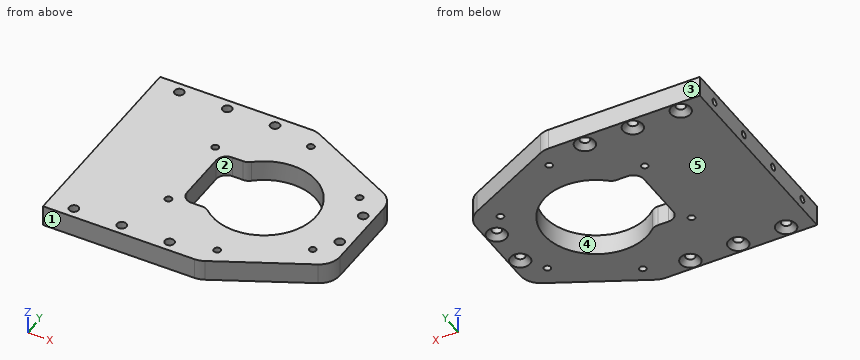
```python
from build123d import *

# Parameters (mm, degrees)
EXTRUDE1_DEPTH                                  = 10
CUT_EXTRUDE1_DEPTH                              = 20
SKETCH3_R                                       = 1.65
CUT_EXTRUDE2_DEPTH                              = 10
SKETCH4_R                                       = 1.65
CUT_EXTRUDE3_DEPTH                              = 15
FILLET1_R                                       = 10
FILLET3_R                                       = 5
SKETCH7_R                                       = 1.5
CUT_EXTRUDE4_DEPTH                              = 10
CSK_FOR_M4_FLAT_HEAD_MACHINE_SCREW2_D           = 4.5
CSK_FOR_M4_FLAT_HEAD_MACHINE_SCREW2_CSINK_D     = 9.4
CSK_FOR_M4_FLAT_HEAD_MACHINE_SCREW2_CSINK_ANGLE = 90
SKETCH10_R                                      = 2.25
CUT_EXTRUDE5_DEPTH                              = 10
CSK_FOR_M4_FLAT_HEAD_MACHINE_SCREW3_D           = 4.5
CSK_FOR_M4_FLAT_HEAD_MACHINE_SCREW3_CSINK_D     = 9.4
CSK_FOR_M4_FLAT_HEAD_MACHINE_SCREW3_CSINK_ANGLE = 90


with BuildPart() as part:
    # Sketch1 → Extrude1 (new body)
    with BuildSketch(Plane.XY):
        Polygon((0, -50), (75, -50), (125, -25), (125, 25), (75, 50), (0, 50), align=None)
    extrude(amount=EXTRUDE1_DEPTH)

    # Sketch2 → Cut-Extrude1 (cut)
    with BuildSketch(Plane.XY.offset(10)):
        with BuildLine():
            Line((60.146428929, -17.5), (48, -17.5))
            Line((48, -17.5), (48, 17.5))
            Line((48, 17.5), (60.146428929, 17.5))
            ThreePointArc((60.146428929, 17.5), (103, 0), (60.146428929, -17.5))
        make_face()
    extrude(amount=-CUT_EXTRUDE1_DEPTH, mode=Mode.SUBTRACT)

    # Sketch3 → Cut-Extrude2 (cut)
    with BuildSketch(Plane(origin=(0, 0, 0), x_dir=(-1, 0, 0), z_dir=(0, 0, -1))):
        with Locations((-112.641016151, 20)):
            Circle(SKETCH3_R)
        with Locations((-78, 40)):
            Circle(SKETCH3_R)
        with Locations((-43.358983849, 20)):
            Circle(SKETCH3_R)
        with Locations((-43.358983849, -20)):
            Circle(SKETCH3_R)
        with Locations((-78, -40)):
            Circle(SKETCH3_R)
        with Locations((-112.641016151, -20)):
            Circle(SKETCH3_R)
    extrude(amount=-CUT_EXTRUDE2_DEPTH, mode=Mode.SUBTRACT)

    # Sketch4 → Cut-Extrude3 (cut)
    with BuildSketch(Plane.ZY):
        with Locations((5, -37.5)):
            Circle(SKETCH4_R)
        with Locations((5, -12.5)):
            Circle(SKETCH4_R)
        with Locations(Location((5, 12.5, 0), (0, 0, 180))):
            Circle(SKETCH4_R)
        with Locations(Location((5, 37.5, 0), (0, 0, 180))):
            Circle(SKETCH4_R)
    extrude(amount=-CUT_EXTRUDE3_DEPTH, mode=Mode.SUBTRACT)

    # Fillet1
    fillet1_edges = [part.edges().sort_by_distance(p)[0] for p in [
        (75, 50, 5),
        (125, 25, 5),
        (125, -25, 5),
        (75, -50, 5),
    ]]
    fillet(fillet1_edges, radius=FILLET1_R)

    # Fillet3
    fillet3_edges = [part.edges().sort_by_distance(p)[0] for p in [
        (60.146428929, 17.5, 5),
        (60.146428929, -17.5, 5),
        (48, -17.5, 5),
        (48, 17.5, 5),
    ]]
    fillet(fillet3_edges, radius=FILLET3_R)

    # Sketch7 → Cut-Extrude4 (cut)
    with BuildSketch(Plane(origin=(0, 0, 0), x_dir=(-1, 0, 0), z_dir=(0, 0, -1))):
        with Locations((-35, -45)):
            Circle(SKETCH7_R)
        with Locations((-12, -45)):
            Circle(SKETCH7_R)
        with Locations(Location((-58, -45, 0), (0, 0, 180))):
            Circle(SKETCH7_R)
        with Locations(Location((-35, 45, 0), (0, 0, 180))):
            Circle(SKETCH7_R)
        with Locations((-58, 45)):
            Circle(SKETCH7_R)
        with Locations(Location((-12, 45, 0), (0, 0, 180))):
            Circle(SKETCH7_R)
    extrude(amount=-CUT_EXTRUDE4_DEPTH, mode=Mode.SUBTRACT)

    # CSK for M4 Flat Head Machine Screw2 (through all)
    with Locations(Plane(origin=(0, 0, 0), x_dir=(-1, 0, 0), z_dir=(0, 0, -1))):
        with Locations((-58, -45), (-35, -45), (-12, -45), (-58, 45), (-35, 45), (-12, 45)):
            CounterSinkHole(CSK_FOR_M4_FLAT_HEAD_MACHINE_SCREW2_D / 2, CSK_FOR_M4_FLAT_HEAD_MACHINE_SCREW2_CSINK_D / 2, counter_sink_angle=CSK_FOR_M4_FLAT_HEAD_MACHINE_SCREW2_CSINK_ANGLE)

    # Sketch10 → Cut-Extrude5 (cut)
    with BuildSketch(Plane(origin=(0, 0, 0), x_dir=(-1, 0, 0), z_dir=(0, 0, -1))):
        with Locations((-120, -10)):
            Circle(SKETCH10_R)
        with Locations(Location((-120, 10, 0), (0, 0, 180))):
            Circle(SKETCH10_R)
    extrude(amount=-CUT_EXTRUDE5_DEPTH, mode=Mode.SUBTRACT)

    # CSK for M4 Flat Head Machine Screw3 (through all)
    with Locations(Plane(origin=(0, 0, 0), x_dir=(-1, 0, 0), z_dir=(0, 0, -1))):
        with Locations((-120, -10), (-120, 10)):
            CounterSinkHole(CSK_FOR_M4_FLAT_HEAD_MACHINE_SCREW3_D / 2, CSK_FOR_M4_FLAT_HEAD_MACHINE_SCREW3_CSINK_D / 2, counter_sink_angle=CSK_FOR_M4_FLAT_HEAD_MACHINE_SCREW3_CSINK_ANGLE)


solid = part.part
```
Check sheet for the modelled part. Datum: model origin and axes. Units: mm. Face numbers are marked on the shaded views. A direction names the side the tool comes from. Give positions to 0.01 mm unless a question says otherwise; leave off trailing zeros. Write each loop counter-clockwise with the first axis right and the second up, starting at its lowest first coordinate (ties: lowest second). Pieces come first, ordered by that corner, then holes. Notation, with made-up numbers: (65.25, 75) - (91.25, 75) arc R23 cw to (91.25, 94) - close; hole circle Ø9 at (71.5, 4.25). An arc over 180 degrees is marked (long way). Answer as a JSON object with one key per item and string values. Group by question number.
1) Depth check by flat-ended pin: P1, Ø2, axis at x = 112.64, y = 20, coming from the -Z side; P2, Ø5.5, axis at x = 112.64, y = -20, coming from the -Z side; P3, Ø1.6, axis at y = 12.5, z = 5.5, coming from the -X side; P4, Ø7, axis at x = 35, y = 45, coming from the -Z side. Enter the tip coordinate at first touch or a pass-through.
2) Release check for a two-part mould opening along Y. For the marked faces 3, 4 and 5 record: pulls with the +Y half, pulls with the -Y half, needs draft (parallel to the pull), parting line crosses it, or undercut.
3) Sectioned sample at C-C (x = 35). Record the cut outline in (y, z).
4) Sectioned sample at D-D (z = 8.5). Give the number of separate pieces and of enclosed holes in the cut face, then the cut area to 3 significant figures.
5) Thickness scan on probe 1 along Y at (x, z) = (53, 1); probe 2 along X at (y, z) = (-9.5, 4.75); probe 3 along X at (y, z) = (-12, 2.5). Record the ranges inside material, lowest first. Write a range as from..to.
6) Access from +Z, -Z, +X, -X, +Y, -Y to the whole of each face (thin tool, end or side, straight path). Record for the marked faces 1 and 2.
7) Sectioned sample at B-B (y = 45). Record the cut outline in (x, z).
8) Sectioned sample at A-A (x = 12). Record the cut outline in (y, z).
Geometry results:
{
 "1": {"P1": "passes through", "P2": "stops at z = 0", "P3": "stops at x = 15", "P4": "stops at z = 1.2"},
 "2": {"face 3": "pulls with the +Y half", "face 4": "undercut", "face 5": "needs draft"},
 "3": {"outline": "(-50, 0) - (-49.7, 0) - (-47.25, 2.45) - (-47.25, 10) - (-50, 10) - close; (-42.75, 2.45) - (-40.3, 0) - (40.3, 0) - (42.75, 2.45) - (42.75, 10) - (-42.75, 10) - close; (47.25, 2.45) - (49.7, 0) - (50, 0) - (50, 10) - (47.25, 10) - close"},
 "4": {"separate pieces": "1", "enclosed holes": "15", "area": "8,850 mm^2"},
 "5": {"probe 1": "y = -50..-17.5, 17.5..50", "probe 2": "x = 0..48, 101.12..117.81, 122.19..125", "probe 3": "x = 0..48, 99.93..118.97, 121.03..125"},
 "6": {"face 1": "+Z, -Z, +X, -X, -Y", "face 2": "+Z, -Z"},
 "7": {"outline": "(0, 0) - (7.3, 0) - (9.75, 2.45) - (9.75, 10) - (0, 10) - close; (14.25, 2.45) - (16.7, 0) - (30.3, 0) - (32.75, 2.45) - (32.75, 10) - (14.25, 10) - close; (37.25, 2.45) - (39.7, 0) - (53.3, 0) - (55.75, 2.45) - (55.75, 10) - (37.25, 10) - close; (60.25, 2.45) - (62.7, 0) - (85, 0) - (85, 10) - (60.25, 10) - close"},
 "8": {"outline": "(-50, 0) - (-49.7, 0) - (-47.25, 2.45) - (-47.25, 10) - (-50, 10) - close; (-42.75, 2.45) - (-40.3, 0) - (40.3, 0) - (42.75, 2.45) - (42.75, 10) - (-42.75, 10) - close; (47.25, 2.45) - (49.7, 0) - (50, 0) - (50, 10) - (47.25, 10) - close; hole circle Ø3.3 at (-37.5, 5); hole circle Ø3.3 at (-12.5, 5); hole circle Ø3.3 at (12.5, 5); hole circle Ø3.3 at (37.5, 5)"}
}
